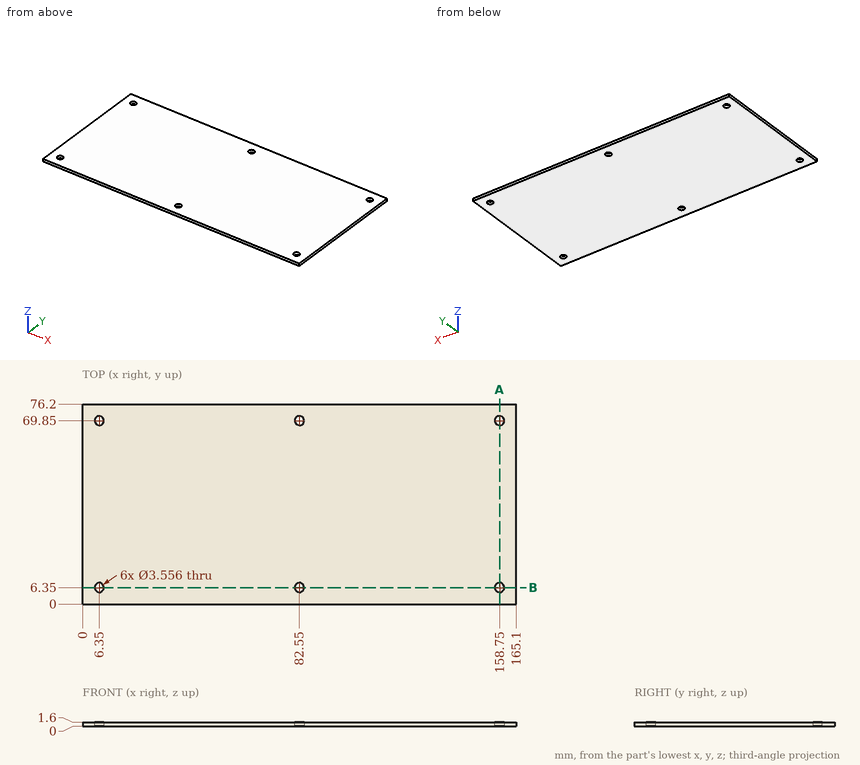
Job drawing, mm, ordinate dimensions from the low corner. One solid piece. Coordinates: 2 decimals unless noted, no trailing zeros. Order: outer loops, then holes, each group sorted by start corner. A loop starts at its lowest first (then second) coordinate and runs counter-clockwise, first axis right, second up. Notation, with made-up numbers: M 40.5,85.25 L 87.5,85.25 A11 ccw 87.5,100.25 Z; hole C -34.75,66 d2. An arc over 180 degrees is marked long. Return JSON: item names as keys, results as strings.
1. Drill centre lines: probe 1 along X at (y, z) = (69.85, 0.8); probe 2 along Y at (x, z) = (158.75, 0.85). Where is each one in solid material? Low to high.
Ans:
{"probe 1": "0 to 4.57, 8.13 to 80.77, 84.33 to 156.97, 160.53 to 165.1", "probe 2": "0 to 4.57, 8.13 to 68.07, 71.63 to 76.2"}
2. Saw through at B-B (y = 6.35). Give the cut face in (x, z), and give its area (3 significant figures).
Ans:
{"outline": "M 0,0 L 4.57,0 L 4.57,1.6 L 0,1.6 Z; M 8.13,0 L 80.77,0 L 80.77,1.6 L 8.13,1.6 Z; M 84.33,0 L 156.97,0 L 156.97,1.6 L 84.33,1.6 Z; M 160.53,0 L 165.1,0 L 165.1,1.6 L 160.53,1.6 Z", "area": "247 mm^2"}
3. Saw through at A-A (x = 158.75). Give the cut face in (y, z).
Ans:
{"outline": "M 0,0 L 4.57,0 L 4.57,1.6 L 0,1.6 Z; M 8.13,0 L 68.07,0 L 68.07,1.6 L 8.13,1.6 Z; M 71.63,0 L 76.2,0 L 76.2,1.6 L 71.63,1.6 Z"}
4. Flat gauge pins, fed straight in: pin 1 (4.5 mm diameter, centred on x = 6.35, y = 69.85, fed in from -Z); pin 2 (2 mm diameter, centred on x = 158.75, y = 69.85, fed in from -Z). Where does each tip first touch, or does it go through?
Ans:
{"pin 1": "z = 0", "pin 2": "through"}
